Here's how the part is built. I have some questions about the finished solid (model axes, mm). Face numbers are marked on the shaded views. A direction names the side the tool comes from. Coordinates: 2 decimals unless noted, no trailing zeros. Write each loop counter-clockwise with the first axis right and the second up, starting at its lowest first coordinate (ties: lowest second). Pieces come first, ordered by that corner, then holes.
Item 1: If we section it at A-A (x = -58): Please give me the cut outline in (y, z).
Item 2: I'm going to push a flat-ended pin straight in: pin 1 Ø5 at (x, y) = (38, -3.5) entering from -Z. Where does the tip first touch, or does it pass through?
Item 3: If I drill on line 1 (Y direction, x = -67.5, z = 28); line 2 (X direction, y = -24.5, z = 2.5); line 3 (Z direction, x = 51, y = -40.5), over which ranges is the centre line in solid material (lowest first)?
Item 4: We'd pull the mould along Y, two halves only. Please class the marked faces 1, 2 and 3: +Y half, -Y half, draft (parallel to the pull), parting line (faces both ways), or undercut.
Item 5: If we section it at C-C (z = 12.25): Please give me the cut outline in (x, y).
Item 6: If we section it at B-B (y = 9.5): Please give me the cut outline in (x, z).
Item 7: If we section it at D-D (x = -18.5): Please give me the cut outline in (y, z), then the cut area to 3 significant figures.
Item 8: For the marked faces 4 and 5, which set-ups out of +Z, -Z, +X, -X, +Y, -Y let a thin tool reach every point of the face, with its end or its side?
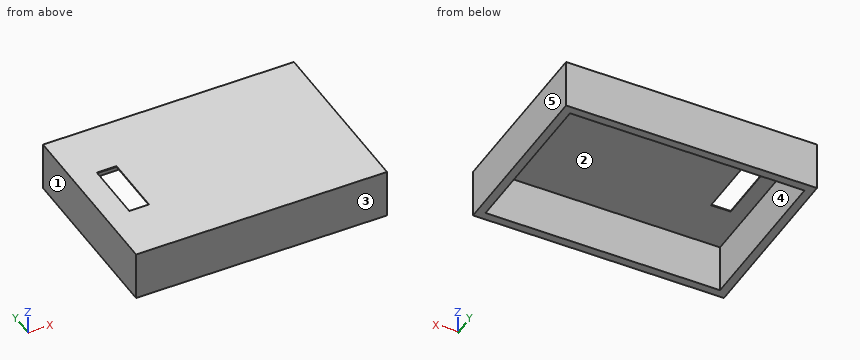
from build123d import *

# Parameters (mm, degrees)
F0_W     = 153
F0_H     = 107.5
F1_DEPTH = 30
F2_W     = 143
F2_H     = 97.5
F3_DEPTH = 29.5


with BuildPart() as f1:
    # F0 (on Top) → F1 (new body)
    with BuildSketch(Plane.XY):
        Rectangle(F0_W, F0_H)
        Polygon((-62.144428, -18.7512), (-62.144428, 18.7488), (-50.144428, 18.7488), (-50.144428, 6.394679), (-50.144428, 0.0036), (-50.144428, -18.7512), align=None, mode=Mode.SUBTRACT)
    extrude(amount=F1_DEPTH)

    # F2 (on Top) → F3 (cut)
    with BuildSketch(Plane.XY):
        Rectangle(F2_W, F2_H)
    extrude(amount=F3_DEPTH, mode=Mode.SUBTRACT)


solid = f1.part
Answer list:
1. outline: (-53.75, 0) - (-48.75, 0) - (-48.75, 29.5) - (-18.75, 29.5) - (-18.75, 30) - (-53.75, 30) - close; (18.75, 29.5) - (48.75, 29.5) - (48.75, 0) - (53.75, 0) - (53.75, 30) - (18.75, 30) - close
2. pin 1: stops at z = 29.5
3. line 1: y = -53.75 to -48.75, 48.75 to 53.75
3. line 2: x = -76.5 to -71.5, 71.5 to 76.5
3. line 3: z = 29.5 to 30
4. face 1: draft
4. face 2: undercut
4. face 3: -Y half
5. outline: (-76.5, -53.75) - (76.5, -53.75) - (76.5, 53.75) - (-76.5, 53.75) - close; hole (-71.5, -48.75) - (71.5, -48.75) - (71.5, 48.75) - (-71.5, 48.75) - close
6. outline: (-76.5, 0) - (-71.5, 0) - (-71.5, 29.5) - (-62.14, 29.5) - (-62.14, 30) - (-76.5, 30) - close; (-50.14, 29.5) - (71.5, 29.5) - (71.5, 0) - (76.5, 0) - (76.5, 30) - (-50.14, 30) - close
7. outline: (-53.75, 0) - (-48.75, 0) - (-48.75, 29.5) - (48.75, 29.5) - (48.75, 0) - (53.75, 0) - (53.75, 30) - (-53.75, 30) - close
7. area: 349 mm2
8. face 4: -Z
8. face 5: +Z, -Z, +X, +Y, -Y
